Model file for the job. Use its own axes, mm. A direction names the side the tool comes from. Give positions to 0.01 mm unless a question says otherwise; leave off trailing zeros. Write each loop counter-clockwise with the first axis right and the second up, starting at its lowest first coordinate (ties: lowest second). Pieces come first, ordered by that corner, then holes.
```python
from build123d import *

# Parameters (mm, degrees)
SKETCH2_R          = 2.6
BASE_FLANGE1_DEPTH = 3
FILLET1_R          = 5
SKETCH3_R          = 2.6
CUT_EXTRUDE1_DEPTH = 10
FILLET2_R          = 2


# Sheet-metal steps are written as plain solids
with BuildPart() as part:
    # Sketch2 → Base-Flange1 (new body)
    with BuildSketch(Plane(origin=(0, 0, 0), x_dir=(1, 0, 0), z_dir=(0, 1, 0))):
        Polygon((0, 60), (32, 60), (50, 50), (50, 0), (20, 0), (20, 20), (0, 20), align=None)
        with Locations(Location((9, 39, 0), (0, 0, 270))):
            Circle(SKETCH2_R, mode=Mode.SUBTRACT)
        with Locations(Location((9, 24, 0), (0, 0, 270))):
            Circle(SKETCH2_R, mode=Mode.SUBTRACT)
        with Locations(Location((28, 9, 0), (0, 0, 270))):
            Circle(SKETCH2_R, mode=Mode.SUBTRACT)
        with Locations(Location((42, 9, 0), (0, 0, 270))):
            Circle(SKETCH2_R, mode=Mode.SUBTRACT)
        with Locations(Location((9, 54, 0), (0, 0, 270))):
            Circle(SKETCH2_R, mode=Mode.SUBTRACT)
    extrude(amount=-BASE_FLANGE1_DEPTH)

    # Fillet1
    fillet1_edges = [part.edges().sort_by_distance(p)[0] for p in [
        (0, -1.5, -20),
        (0, -1.5, -60),
        (32, -1.5, -60),
        (50, -1.5, -50),
        (50, -1.5, 0),
        (20, -1.5, 0),
    ]]
    fillet(fillet1_edges, radius=FILLET1_R)

    # Sketch3 → Cut-Extrude1 (cut)
    with BuildSketch(Plane(origin=(0, 0, 0), x_dir=(1, 0, 0), z_dir=(0, 1, 0))):
        with Locations(Location((45, 35, 0), (0, 0, 270))):
            Circle(SKETCH3_R)
        with Locations(Location((31, 49, 0), (0, 0, 270))):
            Circle(SKETCH3_R)
    extrude(amount=-CUT_EXTRUDE1_DEPTH, mode=Mode.SUBTRACT)

    # Fillet2
    fillet2_edges = [part.edges().sort_by_distance(p)[0] for p in [
        (20, -1.5, -20),
    ]]
    fillet(fillet2_edges, radius=FILLET2_R)


solid = part.part
```
1. Slice it at B-B, the plane x = 41. Write the cut outline in (y, z).
Calculated:
outline: (-3, -55) - (0, -55) - (0, -11.4) - (-3, -11.4) - close; (-3, -6.6) - (0, -6.6) - (0, 0) - (-3, 0) - close
2. Slice it at D-D, the plane y = -0.7. Write the cut outline in (x, z), and give its area (3 significant figures).
Calculated:
outline: (0, -55) arc R5 ccw to (5, -60) - (30.7, -60) arc R5 ccw to (33.13, -59.37) - (47.43, -51.43) arc R5 ccw to (50, -47.06) - (50, -5) arc R5 ccw to (45, 0) - (25, 0) arc R5 ccw to (20, -5) - (20, -18) arc R2 cw to (18, -20) - (5, -20) arc R5 ccw to (0, -25) - close; hole circle Ø5.2 at (9, -54); hole circle Ø5.2 at (9, -39); hole circle Ø5.2 at (9, -24); hole circle Ø5.2 at (28, -9); hole circle Ø5.2 at (31, -49); hole circle Ø5.2 at (42, -9); hole circle Ø5.2 at (45, -35)
area: 2,340 mm2
3. Slice it at C-C, the plane z = -54. Write the cut outline in (x, y).
Calculated:
outline: (0, -3) - (6.4, -3) - (6.4, 0) - (0, 0) - close; (11.6, -3) - (42.8, -3) - (42.8, 0) - (11.6, 0) - close
4. Which spindle directions (+Z, -Z, +X, -X, +Y, -Y) get a long thin tool onto all of the face, cutting with end or side? Do faces 1 (the flat face through (18, -1, -60)), 2 (the flat face through (20, -1, -11)). Say none if no direction does.
Calculated:
face 1: -Z, +X, -X, +Y, -Y
face 2: +Z, -X, +Y, -Y
5. Pull direction Z, two halves, no side cores. Call faces 3 (the flat face through (40.18, -1.479, -55.455)), 4 (the cylindrical face through (6.693, -1.479, -22.8)), 5 (the flat face through (25, 0, -30)): +Z half, -Z half, draft (parallel to the pull), parting line (faces both ways), or undercut.
Calculated:
face 3: -Z half
face 4: undercut
face 5: draft
6. Slice it at A-A, the plane z = -9. Write the cut outline in (x, y).
Calculated:
outline: (20, -3) - (25.4, -3) - (25.4, 0) - (20, 0) - close; (30.6, -3) - (39.4, -3) - (39.4, 0) - (30.6, 0) - close; (44.6, -3) - (50, -3) - (50, 0) - (44.6, 0) - close
7. Probe probe 1 along X at (y, z) = (-0.55, -9); probe 2 along X at (y, z) = (-2.8, -35); probe 3 along Z at (x, y) = (7, -1). List the from-to ranges inside material, lowest first.
Calculated:
probe 1: x = 20 to 25.4, 30.6 to 39.4, 44.6 to 50
probe 2: x = 0 to 42.4, 47.6 to 50
probe 3: z = -60 to -55.66, -52.34 to -40.66, -37.34 to -25.66, -22.34 to -20
